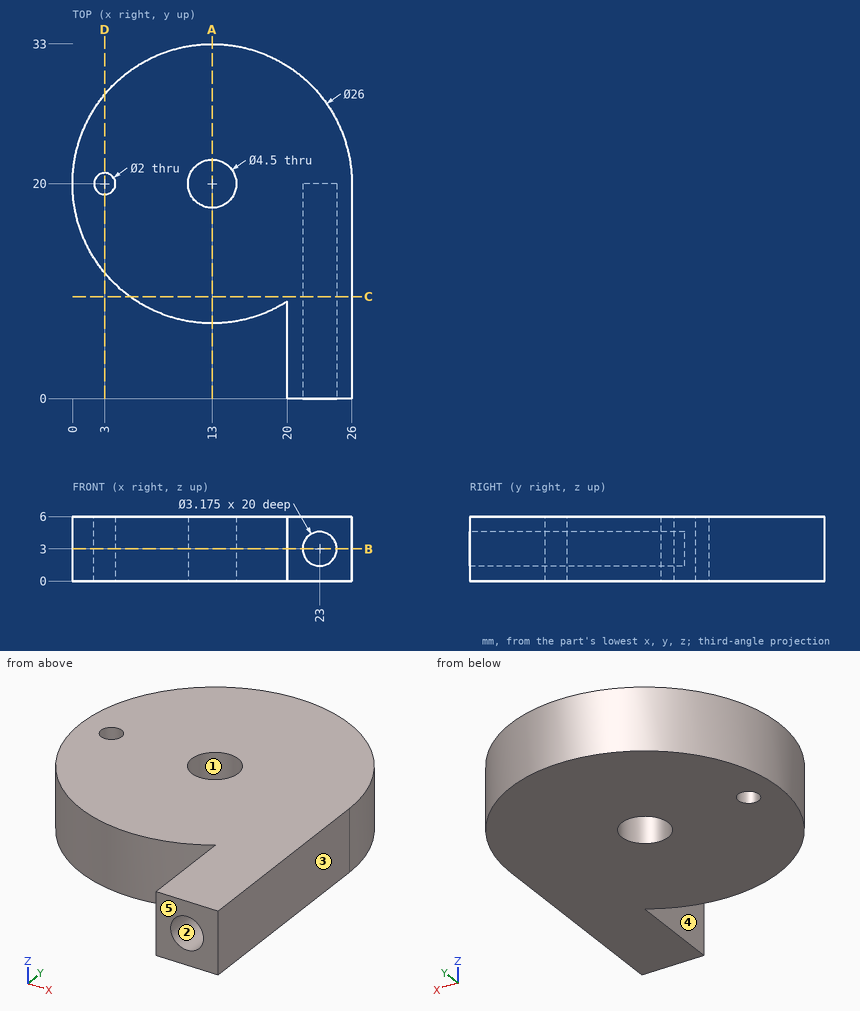
Study the drawing (mm; zero at the part's minimum x, y, z) and answer. A direction names the side the tool comes from. Coordinates: 2 decimals unless noted, no trailing zeros. Write each loop counter-clockwise with the first axis right and the second up, starting at its lowest first coordinate (ties: lowest second). Pieces come first, ordered by that corner, then holes. Notation, with made-up numbers: M 85.5,44 L 132.5,44 A34 cw 132.5,76 Z; hole C 41.25,60.25 d5. An arc over 180 degrees is marked long. Write each question's results on one line, items separated by ' | '.
Item 1: Given P1, Ø2, axis at x = 13.5, z = 3.5, coming from the -Y side; P2, Ø2.5, axis at x = 23, z = 3, coming from the +Y side; P3, Ø3, axis at y = 4.5, z = 4.5, coming from the -X side; P4, Ø2.5, axis at x = 3, y = 20, coming from the +Z side, each flat-ended and moving along its own axis, determine where each tip first touches the part or whether it passes through.
Answer below:
P1: y = 7 | P2: y = 29.61 | P3: x = 20 | P4: z = 6
Item 2: The part is cut by section D-D on x = 3. Determine the outline of the cut face in (y, z).
Answer below:
outline: M 11.69,0 L 19,0 L 19,6 L 11.69,6 Z; M 21,0 L 28.31,0 L 28.31,6 L 21,6 Z
Item 3: The part is cut by section A-A on x = 13. Determine the outline of the cut face in (y, z).
Answer below:
outline: M 7,0 L 17.75,0 L 17.75,6 L 7,6 Z; M 22.25,0 L 33,0 L 33,6 L 22.25,6 Z
Item 4: The part is cut by section B-B on z = 3. Determine the outline of the cut face in (x, y).
Answer below:
outline: M 20,0 L 21.41,0 L 21.41,20 L 24.59,20 L 24.59,0 L 26,0 L 26,20 A13 ccw long 20,9.05 Z; hole C 3,20 d2; hole C 13,20 d4.5
Item 5: The part is cut by section C-C on y = 9.5. Determine the outline of the cut face in (x, z) (1 decimal).
Answer below:
outline: M 5.3,0 L 26,0 L 26,6 L 5.3,6 Z; hole C 23,3 d3.2
Item 6: Consider probe 1 along Y at (x, z) = (13, 3.3); probe 2 along X at (y, z) = (4.5, 3); probe 3 along Z at (x, y) = (23, 15.75). Determine where each line is inside the solid, lowest interval first. Write a range as [from, to].
Answer below:
probe 1: [7, 17.75], [22.25, 33] | probe 2: [20, 21.41], [24.59, 26] | probe 3: [0, 1.41], [4.59, 6]
Item 7: For a pull along X with two mould halves and no side action, classify the marked faces 3, 4 and 5 as released by +X, released by -X, zero draft, split by the parting line, or undercut.
Answer below:
face 3: released by +X | face 4: undercut | face 5: zero draft
Item 8: Which of the six approach directions +Z, -Z, +X, -X, +Y, -Y give full straight-line access (tool end or side, diameter ignored) to the marked faces 1 and 2?
Answer below:
face 1: +Z, -Z | face 2: -Y
